```python
from build123d import *

# Parameters (mm, degrees)
SKETCH1_R           = 12.5
SKETCH1_R_2         = 1.5
BOSS_EXTRUDE1_DEPTH = 4
SKETCH2_R           = 5
BOSS_EXTRUDE2_DEPTH = 3
SKETCH3_R           = 25
BOSS_EXTRUDE3_DEPTH = 20
SKETCH4_R           = 1.5
CUT_EXTRUDE1_DEPTH  = 1.5
SKETCH5_R           = 2
BOSS_EXTRUDE4_DEPTH = 5
SKETCH6_R           = 5.5
CUT_EXTRUDE2_DEPTH  = 1.5
SKETCH7_R           = 1.5
CUT_EXTRUDE3_DEPTH  = 5


with BuildPart() as part:
    # Sketch1 → Boss-Extrude1 (new body)
    with BuildSketch(Plane(origin=(0, 0, 0), x_dir=(0, 1, 0), z_dir=(0, 0, 1))):
        with Locations(Location((0, 0, 0), (0, 0, 270))):
            Circle(SKETCH1_R)
        with Locations(Location((0, 9.5, 0), (0, 0, 270))):
            Circle(SKETCH1_R_2, mode=Mode.SUBTRACT)
        with Locations(Location((-8, 0, 0), (0, 0, 270))):
            Circle(SKETCH1_R_2, mode=Mode.SUBTRACT)
        with Locations(Location((8, 0, 0), (0, 0, 270))):
            Circle(SKETCH1_R_2, mode=Mode.SUBTRACT)
        with Locations(Location((0, -9.5, 0), (0, 0, 270))):
            Circle(SKETCH1_R_2, mode=Mode.SUBTRACT)
    extrude(amount=BOSS_EXTRUDE1_DEPTH)

    # Sketch2 → Boss-Extrude2 (add)
    with BuildSketch(Plane.XY.offset(4)):
        Circle(SKETCH2_R)
    extrude(amount=BOSS_EXTRUDE2_DEPTH)

    # Sketch3 → Boss-Extrude3 (add)
    with BuildSketch(Plane.XY.offset(7)):
        Circle(SKETCH3_R)
    extrude(amount=BOSS_EXTRUDE3_DEPTH)

    # Sketch4 → Cut-Extrude1 (cut, symmetric)
    with BuildSketch(Plane.XY.offset(27)):
        with Locations((0, 6)):
            Circle(SKETCH4_R)
        with Locations((6, 0)):
            Circle(SKETCH4_R)
        with Locations((0, -6)):
            Circle(SKETCH4_R)
        with Locations((-6, 0)):
            Circle(SKETCH4_R)
    extrude(amount=CUT_EXTRUDE1_DEPTH, both=True, mode=Mode.SUBTRACT)

    # Sketch5 → Boss-Extrude4 (add)
    with BuildSketch(Plane.XY.offset(27)):
        Circle(SKETCH5_R)
    extrude(amount=BOSS_EXTRUDE4_DEPTH)

    # Sketch6 → Cut-Extrude2 (cut, symmetric)
    with BuildSketch(Plane(origin=(0, 0, 0), x_dir=(1, 0, 0), z_dir=(0, 0, -1))):
        with Locations(Location((0, 0, 0), (0, 0, 180))):
            Circle(SKETCH6_R)
    extrude(amount=CUT_EXTRUDE2_DEPTH, both=True, mode=Mode.SUBTRACT)

    # Sketch7 → Cut-Extrude3 (cut)
    with BuildSketch(Plane(origin=(0, 0, 1.5), x_dir=(1, 0, 0), z_dir=(0, 0, -1))):
        with Locations(Location((0, 0, 0), (0, 0, 180))):
            Circle(SKETCH7_R)
    extrude(amount=-CUT_EXTRUDE3_DEPTH, mode=Mode.SUBTRACT)


solid = part.part
```
Check sheet for the modelled part. Datum: model origin and axes. Units: mm. A direction names the side the tool comes from. Coordinates: 2 decimals unless noted, no trailing zeros. Order: outer loops, then holes, each group sorted by start corner. A loop starts at its lowest first (then second) coordinate and runs counter-clockwise, first axis right, second up. Notation, with made-up numbers: (34.5, 22.5) -> (75.5, 22.5) arc R28 cw to (75.5, 57.5) -> close; hole circle Ø7 at (29, 30.25). An arc over 180 degrees is marked (long way). Write item = value, one per line. Start each with the question number.
1) Access from +Z, -Z, +X, -X, +Y, -Y to the whole of each face (thin tool, end or side, straight path). Record for faces 4 (the cylindrical face through (-0.325, 6.536, 1.972)), 5 (the flat face through (-0.2, -5.4, 4)), 6 (the flat face through (-6, 0, 0)), 7 (the flat face through (0, 0, 32)), 8 (the cylindrical face through (0, -2, 29)).
2) Cross-section at D-D (z = 16). Enter the section's corners in (x, y), then the cut area to 3 significant figures.
3) Cross-section at C-C (y = 0). State how many separate pieces and enclosed holes the cut face has, then the cut area to 3 significant figures.
4) Cross-section at A-A (x = 9.5). Enter the section's corners in (y, z), then the cut area to 3 significant figures.
5) Mould release check, pull along X, two halves, no side actions. Record for faces 1 (the cylindrical face through (11.923, 3.755, 1.972)), 2 (the flat face through (5, -5, 27)), 3 (the cylindrical face through (-11, 0, 2)): +X half, -X half, draft (parallel to the pull), parting line (faces both ways), or undercut.
6) Go/stop test with flat-tipped pins: P1, Ø12, axis at x = -13, y = 13, coming from the +Z side; P2, Ø0.9, axis at x = -0.5, y = -0.5, coming from the -Z side; P3, Ø1.5, axis at x = 0, y = -6.5, coming from the +Z side; P4, Ø1, axis at x = -14.5, z = 28, coming from the -Y side. Record where each tip stops, or that it passes through.
7) Material ranges on L1, parallel to Y at x = 0, z = 26.55; L2, parallel to Y at x = 0, z = 2.2; L3, parallel to Z at x = 4.5, y = 10.5, recorded low to high.
8) Cross-section at B-B (y = -10.5). Enter the section's corners in (x, z), then the cut area to 3 significant figures.
Ans:
q1.face_4 = -Z
q1.face_5 = none
q1.face_6 = -Z, +X, -X, +Y, -Y
q1.face_7 = +Z, +X, -X, +Y, -Y
q1.face_8 = +Z
q2.outline = circle Ø50 at (0, 0)
q2.area = 1,960 mm²
q3.separate_pieces = 3
q3.enclosed_holes = 0
q3.area = 1,090 mm²
q4.outline = (-23.12, 7) -> (23.12, 7) -> (23.12, 27) -> (-23.12, 27) -> close; (-8.12, 0) -> (-1.5, 0) -> (-1.5, 4) -> (-8.12, 4) -> close; (1.5, 0) -> (8.12, 0) -> (8.12, 4) -> (1.5, 4) -> close
q4.area = 978 mm²
q5.face_1 = parting line
q5.face_2 = draft
q5.face_3 = undercut
q6.P1 = 27
q6.P2 = 6.5
q6.P3 = 25.5
q6.P4 = through
q7.L1 = -25 to -7.5, -4.5 to 4.5, 7.5 to 25
q7.L2 = -12.5 to -9.5, -6.5 to -1.5, 1.5 to 6.5, 9.5 to 12.5
q7.L3 = 0 to 4, 7 to 27
q8.outline = (-22.69, 7) -> (22.69, 7) -> (22.69, 27) -> (-22.69, 27) -> close; (-6.78, 0) -> (6.78, 0) -> (6.78, 4) -> (-6.78, 4) -> close
q8.area = 962 mm²
